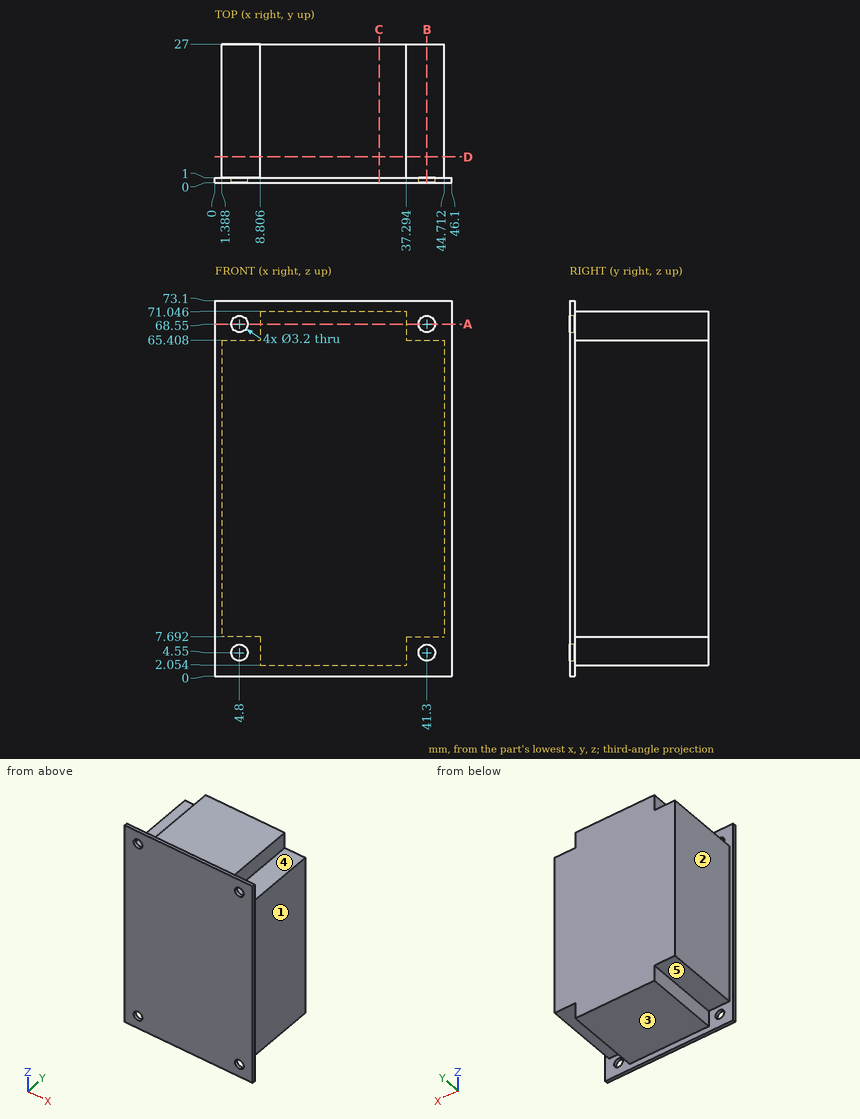
The figure shows three views and two pictorial views of one solid part (mm, origin at its lowest corner). Answer the questions. A direction names the side the tool comes from. Round coordinates to 2 decimals unless told otherwise and drop trailing zeros. Order: outer loops, then holes, each group sorted by start corner. A loop starts at its lowest first (then second) coordinate and runs counter-clockwise, first axis right, second up. Notation, with made-up numbers: (82, 55.5) - (135, 55.5) arc R26 ccw to (135, 72.5) - close; hole circle Ø3 at (67.5, -27.75). An arc over 180 degrees is marked (long way). Write item = value, one per line. Start each with the question number.
1) Section B-B, the plane x = 41.3 is taken. Write down the section's boundary in (y, z).
2) Straight lines are drawn through the part: L1, parallel to X at y = 0.45, z = 4.55; L2, parallel to X at y = 18.25, z = 17; L3, parallel to Z at x = 7, y = 6.75. For each, find the intervals that lie inside material, in ascending order.
3) For the marked faces 1, 2, 3, 4 and 5, determine the directions among +Z, -Z, +X, -X, +Y, -Y from which every point of the face is accessible in a straight line to the end or side of a thin tool.
4) Given pin 1 (5 mm diameter, centred on x = 41.3, z = 4.55, fed in from +Y); pin 2 (2.5 mm diameter, centred on x = 4.8, z = 68.55, fed in from -Y); pin 3 (6 mm diameter, centred on y = 12, z = 41.5, fed in from -X); pin 4 (8 mm diameter, centred on x = 5.5, y = 11, fed in from +Z), each flat-ended and moving along its own axis, determine where each tip first touches the part or whether it passes through.
5) Section C-C, the plane x = 32 is taken. Write down the section's boundary in (y, z) (1 decimal), plus the area to 3 significant figures.
6) Section D-D, the plane y = 5 is taken. Write down the section's boundary in (x, z) (1 decimal), plus the area to 3 significant figures.
7) Section A-A, the plane z = 68.55 is taken. Write down the section's boundary in (x, y).
Results list:
q1.outline = (0, 0) - (1, 0) - (1, 2.95) - (0, 2.95) - close; (0, 6.15) - (1, 6.15) - (1, 7.69) - (27, 7.69) - (27, 65.41) - (1, 65.41) - (1, 66.95) - (0, 66.95) - close; (0, 70.15) - (1, 70.15) - (1, 73.1) - (0, 73.1) - close
q2.L1 = 0 to 3.2, 6.4 to 39.7, 42.9 to 46.1
q2.L2 = 1.39 to 44.71
q2.L3 = 7.69 to 65.41
q3.face_1 = +Z, -Z, +X, +Y
q3.face_2 = +Z, -Z, -X, +Y
q3.face_3 = -Z, +X, -X, +Y
q3.face_4 = +Z, +X, +Y
q3.face_5 = -Z, -X, +Y
q4.pin_1 = 1
q4.pin_2 = through
q4.pin_3 = 1.39
q4.pin_4 = 71.05
q5.outline = (0, 0) - (1, 0) - (1, 2.1) - (27, 2.1) - (27, 71) - (1, 71) - (1, 73.1) - (0, 73.1) - close
q5.area = 1,870 mm^2
q6.outline = (1.4, 7.7) - (8.8, 7.7) - (8.8, 2.1) - (37.3, 2.1) - (37.3, 7.7) - (44.7, 7.7) - (44.7, 65.4) - (37.3, 65.4) - (37.3, 71) - (8.8, 71) - (8.8, 65.4) - (1.4, 65.4) - close
q6.area = 2,820 mm^2
q7.outline = (0, 0) - (3.2, 0) - (3.2, 1) - (0, 1) - close; (6.4, 0) - (39.7, 0) - (39.7, 1) - (37.29, 1) - (37.29, 27) - (8.81, 27) - (8.81, 1) - (6.4, 1) - close; (42.9, 0) - (46.1, 0) - (46.1, 1) - (42.9, 1) - close
